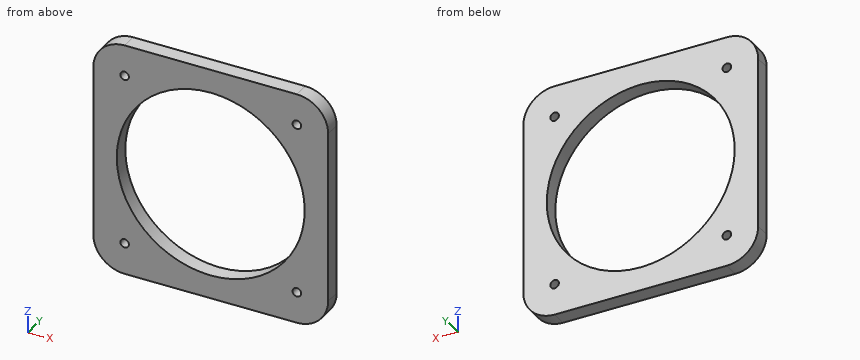
```python
from build123d import *

# Parameters (mm, degrees)
SKETCH1_W           = 95.25
SKETCH1_H           = 95.25
SKETCH1_R           = 38.1
BOSS_EXTRUDE1_DEPTH = 6.35
SKETCH2_R           = 1.75
CUT_EXTRUDE1_DEPTH  = 7.35
CIRPATTERN1_COUNT   = 4
FILLET1_R           = 12.7


with BuildPart() as part:
    # Sketch1 → Boss-Extrude1 (new body)
    with BuildSketch(Plane(origin=(0, 0, 0), x_dir=(1, 0, 0), z_dir=(0, 1, 0))):
        Rectangle(SKETCH1_W, SKETCH1_H)
        Circle(SKETCH1_R, mode=Mode.SUBTRACT)
    extrude(amount=BOSS_EXTRUDE1_DEPTH)

    # Sketch2 → Cut-Extrude1 (cut, through all)
    with BuildSketch(Plane(origin=(0, 6.35, 0), x_dir=(1, 0, 0), z_dir=(0, 1, 0))):
        with Locations((-34.925, 34.925)):
            Circle(SKETCH2_R)
    cut_extrude1 = extrude(amount=-CUT_EXTRUDE1_DEPTH, mode=Mode.SUBTRACT)

    # CirPattern1: Cut-Extrude1 ×4 about axis
    cirpattern1_axis = Axis((0, 0, 0), (0, 1, 0))
    for i in range(1, CIRPATTERN1_COUNT):
        add(cut_extrude1.rotate(cirpattern1_axis, i * 360 / CIRPATTERN1_COUNT), mode=Mode.SUBTRACT)

    # Fillet1
    fillet1_edges = [part.edges().sort_by_distance(p)[0] for p in [
        (-47.625, 3.175, -47.625),
        (47.625, 3.175, -47.625),
        (47.625, 3.175, 47.625),
        (-47.625, 3.175, 47.625),
    ]]
    fillet(fillet1_edges, radius=FILLET1_R)


solid = part.part
```
For this review, take the finished solid that the model builds, in its own axes (mm). Coordinates: 2 decimals unless noted, no trailing zeros. Loops run counter-clockwise (first coordinate to the right, second up) from the corner with the lowest first, then second, coordinate; pieces in that order, holes last. Notation, with made-up numbers: (75.5, 31.25) - (98.5, 31.25) arc R14 ccw to (98.5, 37.25) - close; hole circle Ø11 at (48.25, 68). An arc over 180 degrees is marked (long way). Use one line per item in the form item = value. Start each with the question number.
1) Take a section at A-A (x = 0). State the section outline as (y, z) points (3 decimals), plus the area to 3 significant figures.
2) Take a section at D-D (x = 41.5). State the section outline as (y, z) points.
3) Take a section at C-C (y = 4.25). State the section outline as (x, z) points (3 decimals).
4) To check wall thickness, follow probe 1 along Z at (x, y) = (-34.5, 0.5) (3 decimals); probe 2 along X at (y, z) = (0.5, 5) (1 decimal); probe 3 along Z at (x, y) = (22, 2.25) (3 decimals). State the ranges of each line that lie inside material, in increasing order. Write a range as from..to.
5) Take a section at B-B (z = 0). State the section outline as (x, y) points (3 decimals), plus the area to 3 significant figures.
6) For pin 1 (8 mm diameter, centred on x = -35.5, z = 36.5, fed in from -Y), flat-tipped, find the tip position at first contact; note if it passes through.
From the geometry:
q1.outline = (0, -47.625) - (6.35, -47.625) - (6.35, -38.1) - (0, -38.1) - close; (0, 38.1) - (6.35, 38.1) - (6.35, 47.625) - (0, 47.625) - close
q1.area = 121 mm2
q2.outline = (0, -45.79) - (6.35, -45.79) - (6.35, 45.79) - (0, 45.79) - close
q3.outline = (-47.625, -34.925) arc R12.7 ccw to (-34.925, -47.625) - (34.925, -47.625) arc R12.7 ccw to (47.625, -34.925) - (47.625, 34.925) arc R12.7 ccw to (34.925, 47.625) - (-34.925, 47.625) arc R12.7 ccw to (-47.625, 34.925) - close; hole circle Ø76.2 at (0, 0); hole circle Ø3.5 at (-34.925, -34.925); hole circle Ø3.5 at (-34.925, 34.925); hole circle Ø3.5 at (34.925, -34.925); hole circle Ø3.5 at (34.925, 34.925)
q4.probe_1 = -47.625..-36.623, -33.227..-16.167, 16.167..33.227, 36.623..47.625
q4.probe_2 = -47.6..-37.8, 37.8..47.6
q4.probe_3 = -47.625..-31.106, 31.106..47.625
q5.outline = (-47.625, 0) - (-38.1, 0) - (-38.1, 6.35) - (-47.625, 6.35) - close; (38.1, 0) - (47.625, 0) - (47.625, 6.35) - (38.1, 6.35) - close
q5.area = 121 mm2
q6.pin_1 = 0
